Work out the finished part from the listing and answer in its coordinate system (mm). A direction names the side the tool comes from. Round coordinates to 2 decimals unless told otherwise and drop trailing zeros. Order: outer loops, then holes, each group sorted by start corner. A loop starts at its lowest first (then second) coordinate and runs counter-clockwise, first axis right, second up. Notation, with made-up numbers: M 44,54.5 L 53,54.5 A26 ccw 53,78.5 Z; hole C -4,-23.75 d5. An arc over 180 degrees is marked long. Answer as a JSON object with one key per item and string values. Group by question number.
from build123d import *

# Parameters (mm, degrees)
ESQUISSE1_W             = 140
ESQUISSE1_H             = 100
ESQUISSE1_R             = 4.25
ESQUISSE1_R_2           = 9.151639609
BOSS_EXTRU_1_DEPTH      = 10
ESQUISSE2_W             = 49.107036246
ESQUISSE2_H             = 51.344503494
ESQUISSE2_W_2           = 39.107036246
ESQUISSE2_H_2           = 41.344503494
BOSS_EXTRU_2_DEPTH      = 40
ESQUISSE3_W             = 21.709616914
ESQUISSE3_H             = 34.834623488
ESQUISSE3_W_2           = 19.469502637
ESQUISSE3_H_2           = 23.889605939
BOSS_EXTRU_3_DEPTH      = 30
ESQUISSE4_R             = 6.609240876
ESQUISSE4_R_2           = 6.031853903
ESQUISSE4_R_3           = 6.937899237
ENL_V_MAT_EXTRU_1_DEPTH = 106.095641788


with BuildPart() as part:
    # Esquisse1 → Boss.-Extru.1 (new body)
    with BuildSketch(Plane.XY):
        Rectangle(ESQUISSE1_W, ESQUISSE1_H)
        with Locations((-40, 0)):
            Circle(ESQUISSE1_R, mode=Mode.SUBTRACT)
        with Locations(Location((40, 0, 0), (0, 0, 180))):
            Circle(ESQUISSE1_R, mode=Mode.SUBTRACT)
        Circle(ESQUISSE1_R_2, mode=Mode.SUBTRACT)
    extrude(amount=BOSS_EXTRU_1_DEPTH)

    # Esquisse2 → Boss.-Extru.2 (add)
    with BuildSketch(Plane(origin=(0, 0, 0), x_dir=(-1, 0, 0), z_dir=(0, 0, -1))):
        Rectangle(ESQUISSE2_W, ESQUISSE2_H)
        Rectangle(ESQUISSE2_W_2, ESQUISSE2_H_2, mode=Mode.SUBTRACT)
    extrude(amount=BOSS_EXTRU_2_DEPTH)

    # Esquisse3 → Boss.-Extru.3 (add)
    with BuildSketch(Plane.XY.offset(10)):
        with Locations((-59.145191543, 0)):
            Rectangle(ESQUISSE3_W, ESQUISSE3_H)
        with Locations((59.145191543, 0)):
            Rectangle(ESQUISSE3_W, ESQUISSE3_H)
        with Locations((-22.784580114, 0.210481109)):
            Rectangle(ESQUISSE3_W_2, ESQUISSE3_H_2)
    extrude(amount=BOSS_EXTRU_3_DEPTH)

    # Esquisse4 → Enlèv. mat.-Extru.1 (cut, through all)
    with BuildSketch(Plane(origin=(0, 17.417311744, 0), x_dir=(1, 0, 0), z_dir=(0, 1, 0))):
        with Locations(Location((-59.881875423, -23.83698556, 0), (0, 0, 270))):
            Circle(ESQUISSE4_R)
        with Locations(Location((-22.731959739, -23.83698556, 0), (0, 0, 270))):
            Circle(ESQUISSE4_R_2)
        with Locations(Location((59.671394315, -23.83698556, 0), (0, 0, 270))):
            Circle(ESQUISSE4_R_3)
    extrude(amount=-ENL_V_MAT_EXTRU_1_DEPTH, mode=Mode.SUBTRACT)


solid = part.part
Item 1: Each of these flat-tipped pins is pushed along its axis until it touches: pin 1 (20 mm diameter, centred on x = -2, z = -12.5, fed in from -Y); pin 2 (4 mm diameter, centred on x = 10, z = 13, fed in from -Y); pin 3 (24 mm diameter, centred on x = 57, z = 32, fed in from -Y); pin 4 (19.5 mm diameter, centred on x = -6.5, z = -17, fed in from +Y). Where does it stop, or does it pass through?
Item 2: A tool of negligible diameter and unlimited length cuts with its end or side. For faces 5 (the flat face through (19.554, 0, -20)), 6 (the flat face through (-48.29, 0, 25)), 7 (the flat face through (0, -25.672, -20)), 8 (the flat face through (59, 17.417, 31)), from which of +Z, -Z, +X, -X, +Y, -Y can it reach the whole face along a straight path? Write none if from no direction.
Item 3: Consider L1, parallel to X at y = -1, z = 35.5; L2, parallel to X at y = -17.5, z = -2.5; L3, parallel to Y at x = -15.5, z = -30. Determine where each line is inside the solid, lowest interval first.
Item 4: Find section A-A (x = 0). Give the vertices of the cut face in (y, z), and give its area (3 significant figures).
Item 5: Find section B-B (z = 13.5). Give the vertices of the cut face in (x, y).
Item 6: Find section D-D (y = 23.5). Give the vertices of the cut face in (x, z), and give its area (3 significant figures).
Item 7: Find section C-C (z = 3). Give the vertices of the cut face in (x, y).
Item 8: The mould has two halves that part along Y. Classify faces 1 (the flat face through (-70, -1, 15)), 2 (the flat face through (-1, -50, 5)), 3 (the flat face through (-0.3, 9.5, 0)), 4 (the flat face through (0, 20.672, -20)): +Y half, -Y half, draft (parallel to the pull), parting line (faces both ways), or undercut.
Responses:
{
 "1": {"pin 1": "stops at y = -25.67", "pin 2": "passes through", "pin 3": "stops at y = -17.42", "pin 4": "stops at y = 25.67"},
 "2": {"face 5": "-Z", "face 6": "+Z, +Y, -Y", "face 7": "-Z, +X, -X, -Y", "face 8": "+Z, +X, -X, +Y"},
 "3": {"L1": "x = -70 to -48.29, -32.52 to -13.05, 48.29 to 70", "L2": "x = -24.55 to -19.55, 19.55 to 24.55", "L3": "y = -25.67 to -20.67, 20.67 to 25.67"},
 "4": {"outline": "M -50,0 L -25.67,0 L -25.67,-40 L -20.67,-40 L -20.67,0 L -9.15,0 L -9.15,10 L -50,10 Z; M 9.15,0 L 20.67,0 L 20.67,-40 L 25.67,-40 L 25.67,0 L 50,0 L 50,10 L 9.15,10 Z", "area": "1,220 mm^2"},
 "5": {"outline": "M -70,-17.42 L -48.29,-17.42 L -48.29,17.42 L -70,17.42 Z; M -32.52,-11.73 L -13.05,-11.73 L -13.05,12.16 L -32.52,12.16 Z; M 48.29,-17.42 L 70,-17.42 L 70,17.42 L 48.29,17.42 Z"},
 "6": {"outline": "M -70,0 L -24.55,0 L -24.55,-40 L 24.55,-40 L 24.55,0 L 70,0 L 70,10 L -70,10 Z", "area": "3,360 mm^2"},
 "7": {"outline": "M -70,-50 L 70,-50 L 70,50 L -70,50 Z; hole C -40,0 d8.5; hole C 0,0 d18.3; hole C 40,0 d8.5"},
 "8": {"face 1": "draft", "face 2": "-Y half", "face 3": "undercut", "face 4": "undercut"}
}
